```python
from build123d import *

# Parameters (mm, degrees)
F1_W     = 54.708
F1_H     = 77.4
F2_DEPTH = 1.5
F3_R     = 1.75
F4_DEPTH = 1.5
F5_W     = 20.2
F5_H     = 17.5
F6_DEPTH = 1.501


with BuildPart() as f2:
    # F1 (on face) → F2 (new body)
    with BuildSketch(Plane.XY):
        with Locations((25.654, 37)):
            Rectangle(F1_W, F1_H)
    extrude(amount=F2_DEPTH)

    # F3 (on face) → F4 (join)
    with BuildSketch(Plane(origin=(0, 0, 0), x_dir=(1, 0, 0), z_dir=(0, 0, -1))):
        with BuildLine():
            Line((-1.7, 1.7), (-6.7, 1.7))
            ThreePointArc((-6.7, 1.7), (-11.7, -3.3), (-6.7, -8.3))
            Line((-6.7, -8.3), (-1.7, -8.3))
            Line((-1.7, -8.3), (-1.7, 1.7))
        make_face()
        with Locations((-6.7, -3.3)):
            Circle(F3_R, mode=Mode.SUBTRACT)
        with BuildLine():
            Line((-1.7, -75.7), (-1.7, -80.7))
            ThreePointArc((-1.7, -80.7), (3.3, -85.7), (8.3, -80.7))
            Line((8.3, -80.7), (8.3, -75.7))
            Line((8.3, -75.7), (-1.7, -75.7))
        make_face()
        with Locations((3.3, -80.7)):
            Circle(F3_R, mode=Mode.SUBTRACT)
        with BuildLine():
            Line((53.008, -8.3), (58.008, -8.3))
            ThreePointArc((58.008, -8.3), (63.008, -3.3), (58.008, 1.7))
            Line((58.008, 1.7), (53.008, 1.7))
            Line((53.008, 1.7), (53.008, -8.3))
        make_face()
        with Locations((58.008, -3.3)):
            Circle(F3_R, mode=Mode.SUBTRACT)
        with BuildLine():
            Line((43.008, -75.7), (43.008, -80.7))
            ThreePointArc((43.008, -80.7), (48.008, -85.7), (53.008, -80.7))
            Line((53.008, -80.7), (53.008, -75.7))
            Line((53.008, -75.7), (43.008, -75.7))
        make_face()
        with Locations((48.008, -80.7)):
            Circle(F3_R, mode=Mode.SUBTRACT)
    extrude(amount=-F4_DEPTH)

    # F5 (on face) → F6 (cut, through all)
    with BuildSketch(Plane.XY.offset(1.5)):
        with Locations((8.35, 26)):
            Rectangle(F5_W, F5_H)
        with Locations((42.958, 26)):
            Rectangle(F5_W, F5_H)
        with Locations((8.35, 62)):
            Rectangle(F5_W, F5_H)
        with Locations((42.958, 62)):
            Rectangle(F5_W, F5_H)
    extrude(amount=-F6_DEPTH, mode=Mode.SUBTRACT)


solid = f2.part
```
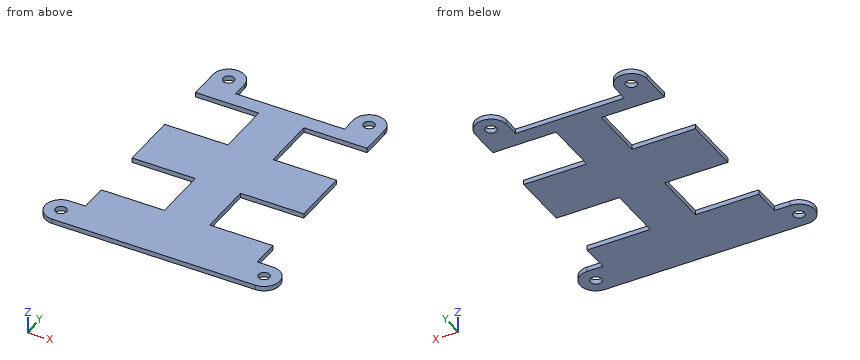
CAD build for the part. Positions are in the model's coordinates, mm. Give positions to 0.01 mm unless a question says otherwise; leave off trailing zeros. Loops run counter-clockwise (first coordinate to the right, second up) from the corner with the lowest first, then second, coordinate; pieces in that order, holes last. Notation, with made-up numbers: (87.25, 52) -> (116.25, 52) arc R4 cw to (116.25, 57) -> close; hole circle Ø9 at (6.5, 87). An arc over 180 degrees is marked (long way). Use a Markdown table: item, result.
1. Slice it at C-C (z = 0.3). Give the number of separate pieces and of enclosed holes in the cut face, plus the area to 3 significant figures.
Check result:
| item | result |
|---|---|
| separate pieces | 1 |
| enclosed holes | 4 |
| area | 3,140 mm^2 |
2. Slice it at B-B (y = 3.3). List the corners of the cut face in (x, z), plus the area to 3 significant figures.
Check result:
| item | result |
|---|---|
| outline | (-11.7, 0) -> (-8.45, 0) -> (-8.45, 1.5) -> (-11.7, 1.5) -> close; (-4.95, 0) -> (56.26, 0) -> (56.26, 1.5) -> (-4.95, 1.5) -> close; (59.76, 0) -> (63.01, 0) -> (63.01, 1.5) -> (59.76, 1.5) -> close |
| area | 102 mm^2 |
3. Slice it at A-A (x = 3.3). List the corners of the cut face in (y, z).
Check result:
| item | result |
|---|---|
| outline | (-1.7, 0) -> (17.25, 0) -> (17.25, 1.5) -> (-1.7, 1.5) -> close; (34.75, 0) -> (53.25, 0) -> (53.25, 1.5) -> (34.75, 1.5) -> close; (70.75, 0) -> (78.95, 0) -> (78.95, 1.5) -> (70.75, 1.5) -> close; (82.45, 0) -> (85.7, 0) -> (85.7, 1.5) -> (82.45, 1.5) -> close |
4. Wall check: L1, parallel to Y at x = 11.5, z = 1.35; L2, parallel to X at y = 80.7, z = 0.4; L3, parallel to X at y = 3.3, z = 0.45. Give the ranges that are in metal, low to high. Write a range as [from, to].
Check result:
| item | result |
|---|---|
| L1 | y = [-1.7, 17.25], [34.75, 53.25], [70.75, 75.7] |
| L2 | x = [-1.7, 1.55], [5.05, 8.3], [43.01, 46.26], [49.76, 53.01] |
| L3 | x = [-11.7, -8.45], [-4.95, 56.26], [59.76, 63.01] |
5. Slice it at D-D (x = 14.5). List the corners of the cut face in (y, z).
Check result:
| item | result |
|---|---|
| outline | (-1.7, 0) -> (17.25, 0) -> (17.25, 1.5) -> (-1.7, 1.5) -> close; (34.75, 0) -> (53.25, 0) -> (53.25, 1.5) -> (34.75, 1.5) -> close; (70.75, 0) -> (75.7, 0) -> (75.7, 1.5) -> (70.75, 1.5) -> close |
6. Flat gauge pins, fed straight in: pin 1 (0.8 mm diameter, centred on y = 79.5, z = 0.5, fed in from -X); pin 2 (0.8 mm diameter, centred on x = 56, z = 1, fed in from +Y); pin 3 (0.8 mm diameter, centred on y = 75, z = 0.5, fed in from +X); pin 4 (3 mm diameter, centred on x = 48.008, y = 80.7, fed in from -Z). Where does each tip first touch, or does it go through?
Check result:
| item | result |
|---|---|
| pin 1 | stops at x = -1.7 |
| pin 2 | stops at y = 8.3 |
| pin 3 | stops at x = 53.01 |
| pin 4 | passes through |
